Check sheet for the drawn part. Datum: minimum x, y, z corner. Units: mm. A direction names the side the tool comes from. Give positions to 0.01 mm unless a question says otherwise; leave off trailing zeros. Loops run counter-clockwise (first coordinate to the right, second up) from the corner with the lowest first, then second, coordinate; pieces in that order, holes last.
1. Go/stop test with flat-tipped pins: pin 1 Ø5.5 at (x, z) = (42.25, 9) entering from -Y; pin 2 Ø2 at (x, y) = (71.5, 26) entering from +Z; pin 3 Ø3.5 at (x, z) = (69.5, 1) entering from +Y; pin 4 Ø0.6 at (x, z) = (48, 4.5) entering from -Y. Record where each tip stops, or that it passes through.
2. Cross-section at B-B, the plane y = 18. Record the cut outline in (x, z), plus the area to 3 significant figures.
3. Cross-section at D-D, the plane x = 74.5. Record the cut outline in (y, z), plus the area to 3 significant figures.
4. Material ranges on L1, parallel to X at y = 31.65, z = 9; L2, parallel to Z at x = 53.25, y = 32.05; L3, parallel to X at y = 18.5, z = 4.5, recorded low to high.
5. Cross-section at C-C, the plane x = 53.25. Record the cut outline in (y, z), plus the area to 3 significant figures.
6. Tool access check on the marked faces 1, 2 and 3. Record the directions out of +Z, -Z, +X, -X, +Y, -Y that give a thin tool (end or side, any length) a straight path to the whole face; none if there is none.
7. Cross-section at A-A, the plane z = 9. Record the cut outline in (x, y), plus the area to 3 significant figures.
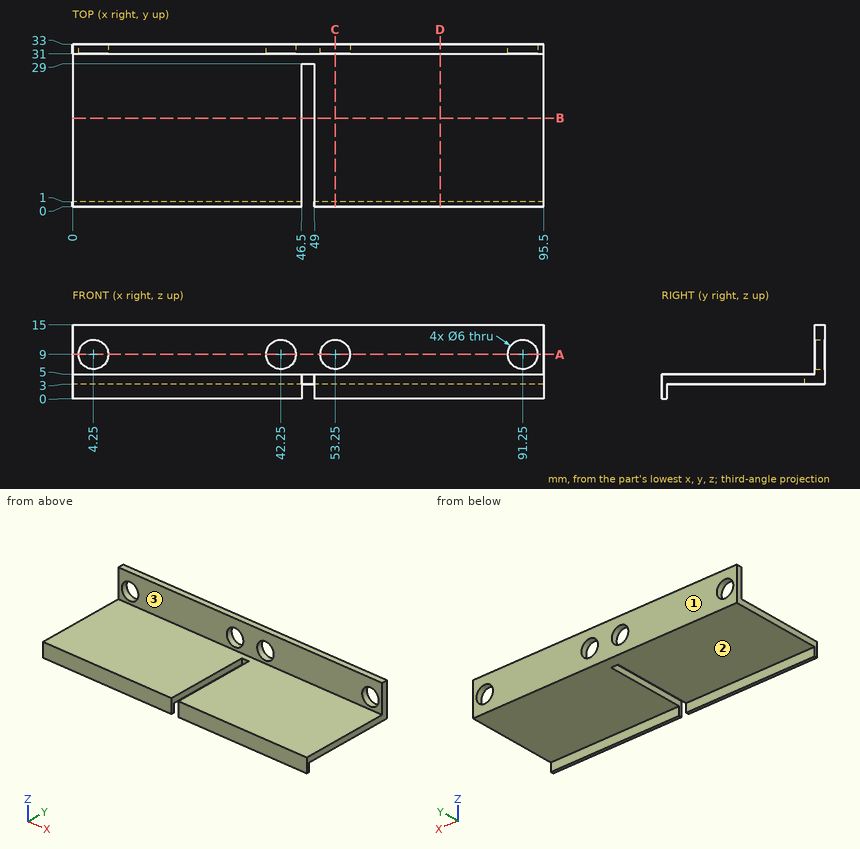
Result:
1. pin 1: passes through
1. pin 2: stops at z = 5
1. pin 3: stops at y = 1
1. pin 4: stops at y = 29
2. outline: (0, 3) - (46.5, 3) - (46.5, 5) - (0, 5) - close; (49, 3) - (95.5, 3) - (95.5, 5) - (49, 5) - close
2. area: 186 mm2
3. outline: (0, 0) - (1, 0) - (1, 3) - (33, 3) - (33, 15) - (31, 15) - (31, 5) - (0, 5) - close
3. area: 89.0 mm2
4. L1: x = 0 to 1.25, 7.25 to 39.25, 45.25 to 50.25, 56.25 to 88.25, 94.25 to 95.5
4. L2: z = 3 to 6, 12 to 15
4. L3: x = 0 to 46.5, 49 to 95.5
5. outline: (0, 0) - (1, 0) - (1, 3) - (33, 3) - (33, 6) - (31, 6) - (31, 5) - (0, 5) - close; (31, 12) - (33, 12) - (33, 15) - (31, 15) - close
5. area: 77.0 mm2
6. face 1: +Z, -Z, +X, -X, +Y
6. face 2: -Z, +X, -X, +Y
6. face 3: +Z, +X, -X, -Y
7. outline: (0, 31) - (1.25, 31) - (1.25, 33) - (0, 33) - close; (7.25, 31) - (39.25, 31) - (39.25, 33) - (7.25, 33) - close; (45.25, 31) - (50.25, 31) - (50.25, 33) - (45.25, 33) - close; (56.25, 31) - (88.25, 31) - (88.25, 33) - (56.25, 33) - close; (94.25, 31) - (95.5, 31) - (95.5, 33) - (94.25, 33) - close
7. area: 143 mm2
